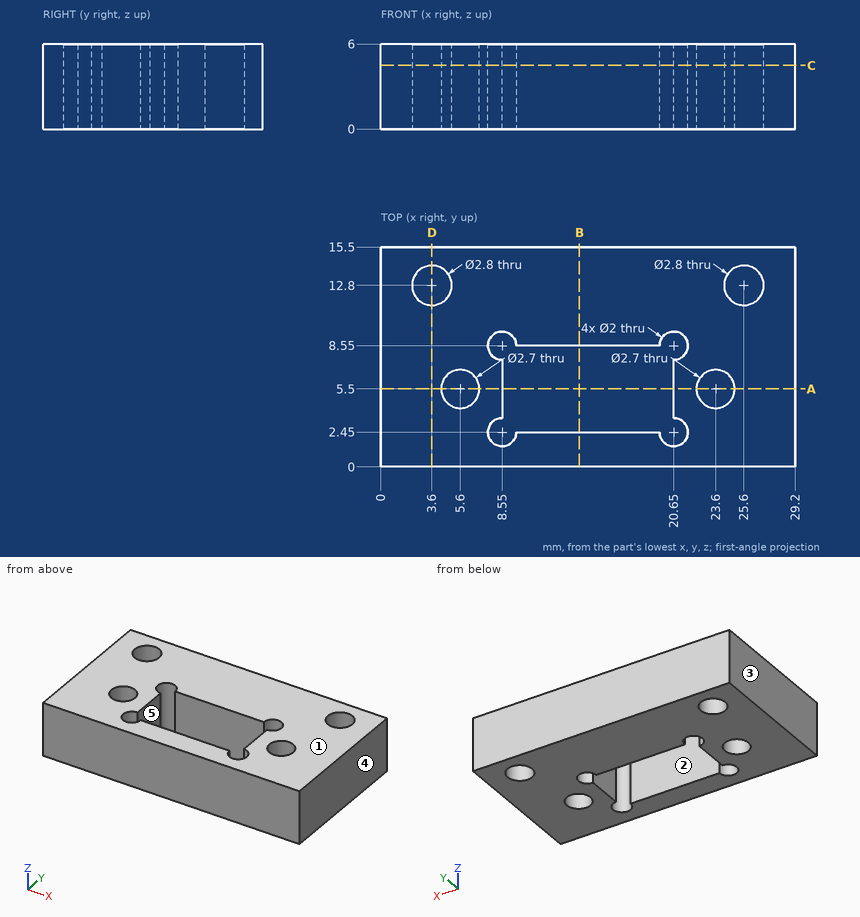
Answer from the drawing. Dimensions are ordinates in mm from the lowest x, y and z of the part. A direction names the side the tool comes from. Coordinates: 2 decimals unless noted, no trailing zeros. Loops run counter-clockwise (first coordinate to the right, second up) from the corner with the lowest first, then second, coordinate; pieces in that order, holes last.
1) Section D-D (x = 3.6) is taken. Give the vertices of the cut face in (y, z), plus the area to 3 significant figures.
Results:
outline: (0, 0) - (11.4, 0) - (11.4, 6) - (0, 6) - close; (14.2, 0) - (15.5, 0) - (15.5, 6) - (14.2, 6) - close
area: 76.2 mm2
2) Section C-C (z = 4.5) is taken. Give the vertices of the cut face in (x, y).
Results:
outline: (0, 0) - (29.2, 0) - (29.2, 15.5) - (0, 15.5) - close; hole circle Ø2.8 at (3.6, 12.8); hole circle Ø2.7 at (5.6, 5.5); hole (8.55, 3.45) arc R1 ccw (long way) to (9.55, 2.45) - (19.65, 2.45) arc R1 ccw (long way) to (20.65, 3.45) - (20.65, 7.55) arc R1 ccw (long way) to (19.65, 8.55) - (9.55, 8.55) arc R1 ccw (long way) to (8.55, 7.55) - close; hole circle Ø2.7 at (23.6, 5.5); hole circle Ø2.8 at (25.6, 12.8)
3) Consider probe 1 along Y at (x, z) = (14, 2); probe 2 along Y at (x, z) = (23.6, 3.75); probe 3 along X at (y, z) = (2.5, 3.95). Determine where each line is inside the solid, lowest interval first.
Results:
probe 1: y = 0 to 2.45, 8.55 to 15.5
probe 2: y = 0 to 4.15, 6.85 to 15.5
probe 3: x = 0 to 7.55, 21.65 to 29.2
4) For a pull along X with two mould halves and no side action, classify the marked faces 1, 2 and 3 as +X half, -X half, draft (parallel to the pull), parting line (faces both ways), or undercut.
Results:
face 1: draft
face 2: undercut
face 3: -X half
5) Section B-B (x = 14) is taken. Give the vertices of the cut face in (y, z), plus the area to 3 significant figures.
Results:
outline: (0, 0) - (2.45, 0) - (2.45, 6) - (0, 6) - close; (8.55, 0) - (15.5, 0) - (15.5, 6) - (8.55, 6) - close
area: 56.4 mm2
6) For the marked faces 4 and 5, determine the directions among +Z, -Z, +X, -X, +Y, -Y from which every point of the face is accessible in a straight line to the end or side of a thin tool.
Results:
face 4: +Z, -Z, +X, +Y, -Y
face 5: +Z, -Z
7) Section A-A (y = 5.5) is taken. Give the vertices of the cut face in (x, z).
Results:
outline: (0, 0) - (4.25, 0) - (4.25, 6) - (0, 6) - close; (6.95, 0) - (8.55, 0) - (8.55, 6) - (6.95, 6) - close; (20.65, 0) - (22.25, 0) - (22.25, 6) - (20.65, 6) - close; (24.95, 0) - (29.2, 0) - (29.2, 6) - (24.95, 6) - close
8) A flat-ended cylindrical pin translates along its axis: pin 1 (1.6 mm diameter, centred on x = 20.65, y = 8.55, fed in from -Z) (3 decimals). Find the tip coordinate at first contact, or state that the pin passes through.
Results:
pin 1: passes through
